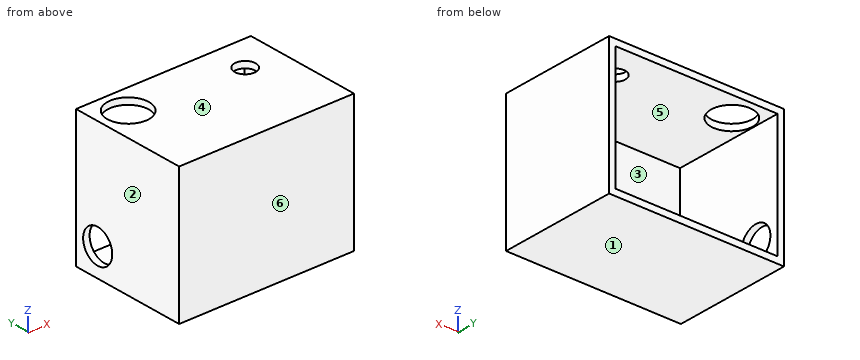
```python
from build123d import *

# Parameters (mm, degrees)
SKETCH1_W           = 85.725
SKETCH1_H           = 66.675
BOSS_EXTRUDE2_DEPTH = 58.42
SHELL1_T            = -3.175
HOLE1_REACH         = 100.466
HOLE1_BORE_R        = 10.16
HOLE2_D             = 16.51
HOLE2_DEPTH         = 3.175
HOLE3_D             = 10.3
HOLE3_DEPTH         = 3.175


with BuildPart() as part:
    # Sketch1 → Boss-Extrude2 (new body)
    with BuildSketch(Plane(origin=(0, 0, 0), x_dir=(1, 0, 0), z_dir=(0, 1, 0))):
        Rectangle(SKETCH1_W, SKETCH1_H)
    extrude(amount=BOSS_EXTRUDE2_DEPTH)

    # Shell1
    shell1_openings = [part.faces().sort_by_distance(p)[0] for p in [
        (0, 58.42, 0),
    ]]
    offset(amount=SHELL1_T, openings=shell1_openings, kind=Kind.INTERSECTION)

    # Hole1 bore → Hole1 (cut, up to next)
    with BuildSketch(Plane.XY.offset(33.3375), mode=Mode.PRIVATE) as hole1_sk1:
        with Locations((-29.033498957, 44.858810897)):
            Circle(HOLE1_BORE_R)
    hole1_tool1 = extrude(hole1_sk1.sketch, amount=-HOLE1_REACH, mode=Mode.PRIVATE) & part.part
    add(hole1_tool1.solids().sort_by_distance((-29.033499, 44.858811, 33.3375))[0], mode=Mode.SUBTRACT)

    # Hole2
    with Locations(Plane.ZY.offset(42.8625)):
        with Locations((-19.658206751, 46.146926064)):
            Hole(HOLE2_D / 2, depth=HOLE2_DEPTH)

    # Hole3
    with Locations(Plane.XY.offset(33.3375)):
        with Locations((25.3625, 41.42)):
            Hole(HOLE3_D / 2, depth=HOLE3_DEPTH)


solid = part.part
```
Geometry check sheet. Reference: the model listing, model coordinates, mm. Face numbers are marked on the shaded views. A direction names the side the tool comes from. Round coordinates to 2 decimals unless told otherwise and drop trailing zeros. Order: outer loops, then holes, each group sorted by start corner. A loop starts at its lowest first (then second) coordinate and runs counter-clockwise, first axis right, second up. Notation, with made-up numbers: (-28, -38.5) - (12, -38.5) arc R32 ccw to (12, -10.5) - close; hole circle Ø3 at (75.25, -0.75). An arc over 180 degrees is marked (long way). Use a Markdown table: item, result. Add a question column.
(1) Tool access check on the marked faces 5 and 6. Record the directions out of +Z, -Z, +X, -X, +Y, -Y that give a thin tool (end or side, any length) a straight path to the whole face; none if there is none.
(2) Sectioned sample at D-D, the plane z = -18. Enter the section's corners in (x, y) (1 decimal).
(3) Sectioned sample at A-A, the plane y = 32. Enter the section's corners in (x, z).
(4) Material ranges on line 1 along Z through (x, y) = (35.5, 33.5); line 2 along X through (y, z) = (6, 22); line 3 along Y through (x, z) = (14, -21.5) (3 decimals), recorded low to high. Write a range as [from, to].
(5) Sectioned sample at B-B, the plane x = -10.5. Enter the section's corners in (y, z) (1 decimal).
(6) Release check for a two-part mould opening along Z. For the marked faces 1, 2, 3 and 4 record: pulls with the +Z half, pulls with the -Z half, needs draft (parallel to the pull), parting line crosses it, or undercut.
(7) Sectioned sample at C-C, the plane z = 3.5. Enter the section's corners in (x, y) (1 decimal), and give its area (3 significant figures).
Answers below:
| question | item | result |
|---|---|---|
| 1 | face 5 | +Y |
| 1 | face 6 | +Z, -Z, +X, -X, -Y |
| 2 | outline | (-42.9, 0) - (42.9, 0) - (42.9, 58.4) - (39.7, 58.4) - (39.7, 3.2) - (-39.7, 3.2) - (-39.7, 38.1) - (-42.9, 38.1) - close; (-42.9, 54.2) - (-39.7, 54.2) - (-39.7, 58.4) - (-42.9, 58.4) - close |
| 3 | outline | (-42.86, -33.34) - (42.86, -33.34) - (42.86, 33.34) - (-42.86, 33.34) - close; hole (-39.69, -30.16) - (39.69, -30.16) - (39.69, 30.16) - (-39.69, 30.16) - close |
| 4 | line 1 | [-33.34, -30.16], [30.16, 33.34] |
| 4 | line 2 | [-42.86, -39.69], [39.69, 42.86] |
| 4 | line 3 | [0, 3.175] |
| 5 | outline | (0, -33.3) - (58.4, -33.3) - (58.4, -30.2) - (3.2, -30.2) - (3.2, 30.2) - (58.4, 30.2) - (58.4, 33.3) - (0, 33.3) - close |
| 6 | face 1 | pulls with the -Z half |
| 6 | face 2 | needs draft |
| 6 | face 3 | undercut |
| 6 | face 4 | pulls with the +Z half |
| 7 | outline | (-42.9, 0) - (42.9, 0) - (42.9, 58.4) - (39.7, 58.4) - (39.7, 3.2) - (-39.7, 3.2) - (-39.7, 58.4) - (-42.9, 58.4) - close |
| 7 | area | 623 mm² |
